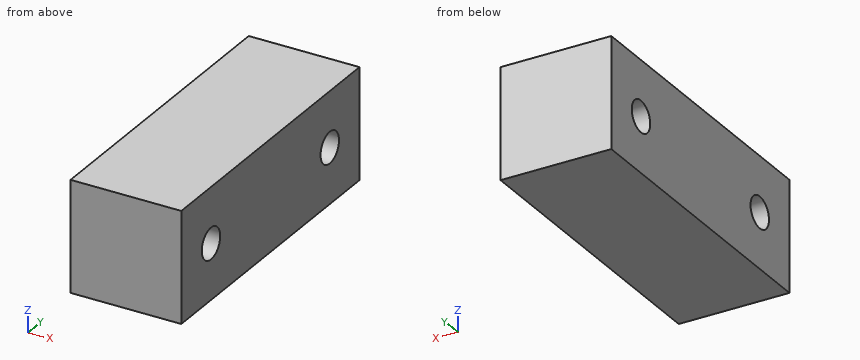
```python
from build123d import *

# Parameters (mm, degrees)
SKETCH1_W           = 13.97
SKETCH1_H           = 38.1
BOSS_EXTRUDE1_DEPTH = 13.97
SKETCH2_R           = 1.9685
CUT_EXTRUDE2_DEPTH  = 13.97


with BuildPart() as part:
    # Sketch1 → Boss-Extrude1 (new body)
    with BuildSketch(Plane.XY):
        with Locations((-37.077191011, -17.498671499)):
            Rectangle(SKETCH1_W, SKETCH1_H)
    extrude(amount=BOSS_EXTRUDE1_DEPTH)

    # Sketch2 → Cut-Extrude2 (cut)
    with BuildSketch(Plane.ZY.offset(44.062191011)):
        with Locations(Location((6.985, -4.798671499, 0), (0, 0, 270))):
            Circle(SKETCH2_R)
        with Locations(Location((6.985, -30.198671499, 0), (0, 0, 270))):
            Circle(SKETCH2_R)
    extrude(amount=-CUT_EXTRUDE2_DEPTH, mode=Mode.SUBTRACT)


solid = part.part
```
Part model, mm, in its own coordinate system. Round coordinates to 2 decimals unless told otherwise and drop trailing zeros. Write each loop counter-clockwise with the first axis right and the second up, starting at its lowest first coordinate (ties: lowest second). Pieces come first, ordered by that corner, then holes. Notation, with made-up numbers: M -30,83 L 17,83 A10 ccw 17,87 Z; hole C 15,-17.5 d11. An arc over 180 degrees is marked long. Answer as CSV lines item,"result". Start each with the question number.
1) Band-saw the part on B-B (x = -37). List the corners of the cut face in (y, z) (1 decimal).
2) Drill centre lines: L1, parallel to Y at x = -34.5, z = 8; L2, parallel to Y at x = -40.5, z = 7; L3, parallel to Z at x = -40.75, y = -3.5. Where is each one in solid material? Low to high.
3) Band-saw the part on A-A (y = -30). List the corners of the cut face in (x, z).
Worked out:
1,outline,"M -36.5,0 L 1.6,0 L 1.6,14 L -36.5,14 Z; hole C -30.2,7 d3.9; hole C -4.8,7 d3.9"
2,L1,"-36.55 to -31.89, -28.51 to -6.49, -3.11 to 1.55"
2,L2,"-36.55 to -32.17, -28.23 to -6.77, -2.83 to 1.55"
2,L3,"0 to 5.51, 8.46 to 13.97"
3,outline,"M -44.06,0 L -30.09,0 L -30.09,5.03 L -44.06,5.03 Z; M -44.06,8.94 L -30.09,8.94 L -30.09,13.97 L -44.06,13.97 Z"
